Model file for the job. Use its own axes, mm. Face numbers are marked on the shaded views. A direction names the side the tool comes from. Give positions to 0.01 mm unless a question says otherwise; leave off trailing zeros. Loops run counter-clockwise (first coordinate to the right, second up) from the corner with the lowest first, then second, coordinate; pieces in that order, holes last. Notation, with made-up numbers: (-19, -35.5) - (34, -35.5) arc R27 ccw to (34, -7.5) - close; hole circle Ø11 at (54.5, 81). An arc over 180 degrees is marked (long way). Answer as CSV lines item,"result". Start each with the question number.
Item 1: Tool access for the marked faces 5 and 6: list every direction of +Z, -Z, +X, -X, +Y, -Y with a clear straight run to the whole face (end or side of a thin tool).
Item 2: Saw through at A-A on y = 20. Give the cut face in (x, z).
Item 3: Saw through at C-C on x = -18. Give the cut face in (y, z).
Item 4: Pull direction Z, two halves, no side cores. Call the marked faces 1, 2, 3 and 4: pulls with the +Z half, pulls with the -Z half, needs draft (parallel to the pull), parting line crosses it, or undercut.
Item 5: Pin check, flat tips, straight feed: pin 1 (5 mm diameter, centred on y = 18, z = -77.5, fed in from +X); pin 2 (2.5 mm diameter, centred on x = -48.935, z = -14.045, fed in from +Y); pin 3 (6.5 mm diameter, centred on x = -116.91, z = -67.5, fed in from +Y). Stop position of each tip, or through.
Item 6: Drill centre lines: L1, parallel to X at y = 5.85, z = -67.5; L2, parallel to X at y = 2.45, z = -2.5; L3, parallel to X at y = 35.5, z = -9. Where is each one in solid material? Low to high. Write a range as from..to.
Item 7: Saw through at B-B on z = -30. Give the cut face in (x, y), plus the area to 3 significant figures.
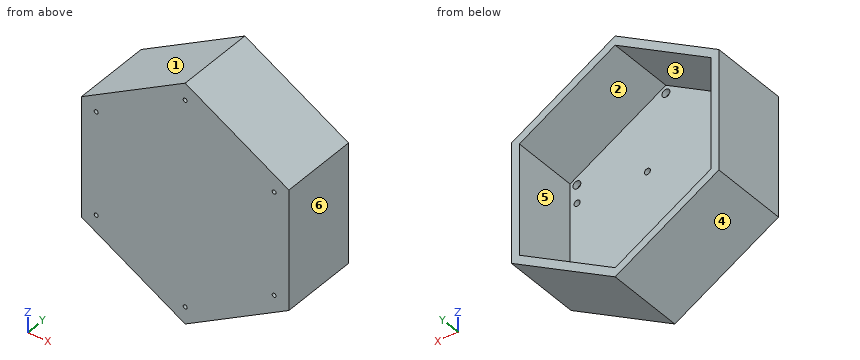
Autodesk Inventor part; units mm, degrees
ref_plane "YZ Plane" through (0, 0, 0) normal (1, 0, 0) x (0, 1, 0)
ref_plane "XZ Plane" through (0, 0, 0) normal (0, 1, 0) x (-1, 0, 0)
ref_plane "XY Plane" through (0, 0, 0) normal (0, 0, 1) x (1, 0, 0)
sketch "Sketch1" plane through (0, 0, 0) normal (0, 1, 0) x (-1, 0, 0)
  line L0 (0, 0) -> (0, -70)
  line L1 (0, -70) -> (60.6218, -105)
  line L2 (60.6218, -105) -> (121.2436, -70)
  line L3 (121.2436, -70) -> (121.2436, 0)
  line L4 (121.2436, 0) -> (60.6218, 35)
  line L5 (60.6218, 35) -> (0, 0)
  line L6 (-5, 2.8868) -> (-5, -72.8868)
  line L7 (-5, -72.8868) -> (60.6218, -110.7735)
  line L8 (60.6218, -110.7735) -> (126.2436, -72.8868)
  line L9 (126.2436, -72.8868) -> (126.2436, 2.8868)
  line L10 (126.2436, 2.8868) -> (60.6218, 40.7735)
  line L11 (60.6218, 40.7735) -> (-5, 2.8868)
  line L12 (0, 0) -> (-5, 0) construction
  line L13 (-5, 2.8868) -> (0, 0) construction
  dimension "wall" = 70
  dimension "d1" = 70
  dimension "d2" = 70
  dimension "d3" = 70
  dimension "d4" = 70
  dimension "d5" = 70
  dimension "d6" = 120
  dimension "d7" = 120
  dimension "d9" = 120
  dimension "d10" = 120
  dimension "d11" = 120
  dimension "wallThickness" = 5
  dimension "d15" = 5
  dimension "d16" = 131.2436
extrude "Extrusion1" add sketch "Sketch1" along normal blind 7.5 contours L5 L4 L3 L2 L1 L0
extrude "Extrusion2" add sketch "Sketch1" along normal blind 50
sketch "Sketch2" plane through (0, 7.5, 0) normal (0, 1, 0) x (1, 0, 0)
  circle A0 centre (-4.45, 55.955) radius 1.905
  circle A1 centre (-4.45, 14.045) radius 1.905
  line L0 (-4.45, 55.955) -> (-4.45, 14.045) construction
  line L1 (0, 70) -> (0, 0) construction
  line L2 (-4.45, 14.045) -> (-48.935, 14.045) construction
  circle A2 centre (-48.935, 14.045) radius 1.905
  circle A3 centre (-48.935, 55.955) radius 1.905
  line L3 (0, 70) -> (-60.6218, 105)
  line L4 (0, 70) -> (-1, 70) construction
  dimension "holderRadius" = 3.81
  dimension "d22" = 3.81
  dimension "d23" = 41.91
  dimension "d24" = 4.45
  dimension "d25" = 44.485
  dimension "d26" = 3.81
  dimension "d27" = 3.81
  dimension "d28" = 41.91
  dimension "d29" = 44.485
  dimension "d30" = 1
  dimension "d31" = 14.045
extrude "Extrusion3" cut sketch "Sketch2" against normal blind 5
sketch "Sketch3" plane through (0, 7.5, 0) normal (0, 1, 0) x (1, 0, 0)
  circle A0 centre (-4.3301, 2.5) radius 2.5
  line L0 (0, 0) -> (0, 70)
  line L1 (0, 0) -> (-4.3301, 2.5) construction
  line L2 (0, 0) -> (5, 0) construction
  line L3 (-60.6218, -35) -> (-121.2436, 0) construction
  line L4 (-60.6218, -35) -> (-60.6218, -30) construction
  line L5 (-60.6218, -35) -> (-55.6218, -35) construction
  line L6 (-121.2436, 70) -> (-121.2436, 0) construction
  line L7 (-121.2436, 0) -> (-116.9134, 2.5) construction
  line L8 (-121.2436, 0) -> (-116.2436, 0) construction
  line L9 (-60.6218, 105) -> (-60.6218, 100) construction
  line L10 (0, 70) -> (-4.3301, 67.5) construction
  circle A1 centre (-4.3301, 67.5) radius 2.5
  line L11 (-121.2436, 70) -> (-60.6218, 105) construction
  circle A2 centre (-116.9134, 2.5) radius 2.5
  line L12 (-121.2436, 70) -> (-116.9134, 67.5) construction
  circle A3 centre (-116.9134, 67.5) radius 2.5
  circle A4 centre (-60.6218, 100) radius 2.5
  circle A5 centre (-60.6218, -30) radius 2.5
  circle A6 centre (-60.6218, -30) radius 1.25
  circle A7 centre (-116.9134, 2.5) radius 1.25
  circle A8 centre (-116.9134, 67.5) radius 1.25
  circle A9 centre (-60.6218, 100) radius 1.25
  circle A10 centre (-4.3301, 67.5) radius 1.25
  circle A11 centre (-4.3301, 2.5) radius 1.25
  dimension "holeRad" = 5
  dimension "d35" = 5
  dimension "d36" = 150
  dimension "d37" = 5
  dimension "d38" = 90
  dimension "d39" = 5
  dimension "d40" = 30
  dimension "d42" = 5
  dimension "d43" = 5
  dimension "d44" = 5
  dimension "d45" = 60
  dimension "d47" = 5
  dimension "d48" = 5
  dimension "d49" = 60
  dimension "d50" = 5
  dimension "d51" = 5
  dimension "d52" = 5
  dimension "d53" = 2.5
  dimension "d54" = 2.5
  dimension "d55" = 2.5
  dimension "d56" = 2.5
  dimension "d57" = 2.5
  dimension "d58" = 2.5
extrude "Extrusion4" cut sketch "Sketch3" against normal blind 3.75
extrude "Extrusion5" cut sketch "Sketch3" against normal blind 7.5 contours A6 | A7 | A8 | A9 | A10 | A11
equation "\"d1\" = wall"
equation "\"d2\" = wall"
equation "\"d3\" = wall"
equation "\"d4\" = wall"
equation "\"d5\" = wall"
properties part number "Improved Internal Base"
Responses:
1,face 5,"+Y"
1,face 6,"+Z, -Z, +X, +Y, -Y"
2,outline,"(-126.24, -72.89) - (-60.62, -110.77) - (5, -72.89) - (5, 2.89) - (-60.62, 40.77) - (-126.24, 2.89) - close; hole (-121.24, -70) - (-60.62, -105) - (0, -70) - (0, 0) - (-60.62, 35) - (-121.24, 0) - close"
3,outline,"(0, -86.17) - (50, -86.17) - (50, -80.39) - (7.5, -80.39) - (7.5, 10.39) - (50, 10.39) - (50, 16.17) - (0, 16.17) - close"
4,face 1,"pulls with the +Z half"
4,face 2,"undercut"
4,face 3,"undercut"
4,face 4,"pulls with the -Z half"
5,pin 1,"x = 1.34"
5,pin 2,"y = 2.5"
5,pin 3,"y = 7.5"
6,L1,"-126.24..-119.41, -114.41..-6.83, -1.83..5"
6,L2,"-126.24..-118.16, -115.66..-5.58, -3.08..5"
6,L3,"-126.24..-121.24, 0..5"
7,outline,"(-126.24, 0) - (5, 0) - (5, 50) - (0, 50) - (0, 7.5) - (-121.24, 7.5) - (-121.24, 50) - (-126.24, 50) - close"
7,area,"1,410 mm2"
